from build123d import *

# Parameters (mm, degrees)
ESQUISSE1_R             = 16.4
BOSS_EXTRU_1_DEPTH      = 2
ESQUISSE3_R             = 3
ENL_V_MAT_EXTRU_1_DEPTH = 3
ESQUISSE4_W             = 72.110421533
ESQUISSE4_H             = 46.707886675
ESQUISSE4_W_2           = 31
ESQUISSE4_H_2           = 31
ENL_V_MAT_EXTRU_2_DEPTH = 10
CONG_1_R                = 10


with BuildPart() as part:
    # Esquisse1 → Boss.-Extru.1 (new body)
    with BuildSketch(Plane.XY):
        Circle(ESQUISSE1_R)
    extrude(amount=BOSS_EXTRU_1_DEPTH)

    # Esquisse3 → Enlèv. mat.-Extru.1 (cut, through all)
    with BuildSketch(Plane.XY.offset(2)):
        Circle(ESQUISSE3_R)
    extrude(amount=-ENL_V_MAT_EXTRU_1_DEPTH, mode=Mode.SUBTRACT)

    # Esquisse4 → Enlèv. mat.-Extru.2 (cut)
    with BuildSketch(Plane(origin=(0, 0, 0), x_dir=(-1, 0, 0), z_dir=(0, 0, -1))):
        with Locations((-0.063033586, -0.977020572)):
            Rectangle(ESQUISSE4_W, ESQUISSE4_H)
        Rectangle(ESQUISSE4_W_2, ESQUISSE4_H_2, mode=Mode.SUBTRACT)
    extrude(amount=-ENL_V_MAT_EXTRU_2_DEPTH, mode=Mode.SUBTRACT)

    # Congé1
    cong_1_edges = [part.edges().sort_by_distance(p)[0] for p in [
        (15.5, -5.35817133, 1),
        (15.5, 5.35817133, 1),
        (5.35817133, 15.5, 1),
        (-5.35817133, 15.5, 1),
        (-15.5, 5.35817133, 1),
        (-15.5, -5.35817133, 1),
        (-5.35817133, -15.5, 1),
        (5.35817133, -15.5, 1),
    ]]
    fillet(cong_1_edges, radius=CONG_1_R)


solid = part.part
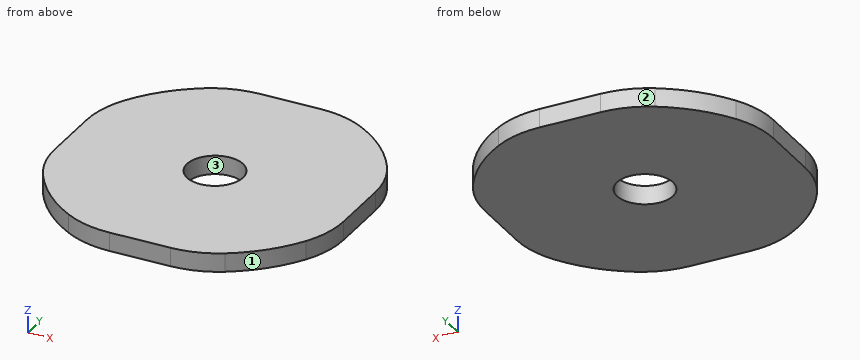
Source: CAD feature listing. Evaluate the final solid. Frame: model axes, mm. Face numbers are marked on the shaded views. Coordinates: 2 decimals unless noted, no trailing zeros. Order: outer loops, then holes, each group sorted by start corner. A loop starts at its lowest first (then second) coordinate and runs counter-clockwise, first axis right, second up.
Item 1: Cut plane A-A (y = 0). Return loops of the section in (x, z), plus the area to 3 significant figures.
Output values:
outline: (-15.5, 0) - (-3, 0) - (-3, 2) - (-15.5, 2) - close; (3, 0) - (15.5, 0) - (15.5, 2) - (3, 2) - close
area: 50.0 mm2
Item 2: Material intervals for line 1 (Y direction, x = 0, z = 1.6); line 2 (X direction, y = 1.5, z = 0.3); line 3 (X direction, y = 3.5, z = 0.7), sorted ascending.
Output values:
line 1: y = -15.5 to -3, 3 to 15.5
line 2: x = -15.5 to -2.6, 2.6 to 15.5
line 3: x = -15.5 to 15.5
Item 3: Cut plane C-C (z = 0.7). Return loops of the section in (x, y), plus the area to 3 significant figures.
Output values:
outline: (-15.5, -3.27) arc R10 ccw to (-14.09, -8.39) arc R16.4 ccw to (-8.39, -14.09) arc R10 ccw to (-3.27, -15.5) - (3.27, -15.5) arc R10 ccw to (8.39, -14.09) arc R16.4 ccw to (14.09, -8.39) arc R10 ccw to (15.5, -3.27) - (15.5, 3.27) arc R10 ccw to (14.09, 8.39) arc R16.4 ccw to (8.39, 14.09) arc R10 ccw to (3.27, 15.5) - (-3.27, 15.5) arc R10 ccw to (-8.39, 14.09) arc R16.4 ccw to (-14.09, 8.39) arc R10 ccw to (-15.5, 3.27) - close; hole circle Ø6 at (0, 0)
area: 788 mm2
Item 4: Pull-direction query (X, two-part tool) for the marked faces 1, 2 and 3; classes: pulls with the +X half, pulls with the -X half, needs draft (parallel to the pull), parting line crosses it, or undercut.
Output values:
face 1: pulls with the +X half
face 2: pulls with the -X half
face 3: undercut
Item 5: Cut plane D-D (x = -8). Return loops of the section in (y, z), plus the area to 3 significant figures.
Output values:
outline: (-14.31, 0) - (14.31, 0) - (14.31, 2) - (-14.31, 2) - close
area: 57.2 mm2
Item 6: First-contact query: P1, Ø1, axis at y = 8.5, z = 0.5, coming from the +X side. Flat tip, straight axial feed; report the tip coordinate or a pass-through.
Output values:
P1: stops at x = 14.31
